Could you check a few things on this model? Use its own coordinates, in mm. Face numbers are marked on the shaded views. A direction names the side the tool comes from. Coordinates: 2 decimals unless noted, no trailing zeros. Write each loop counter-clockwise with the first axis right and the second up, starting at its lowest first coordinate (ties: lowest second). Pieces come first, ordered by that corner, then holes. Notation, with made-up numbers: (66, -7.75) - (111, -7.75) arc R27 ccw to (111, 11.25) - close; hole circle Ø8 at (-21.5, 89). An arc over 180 degrees is marked (long way). Write item = value, one per line. Start each with the question number.
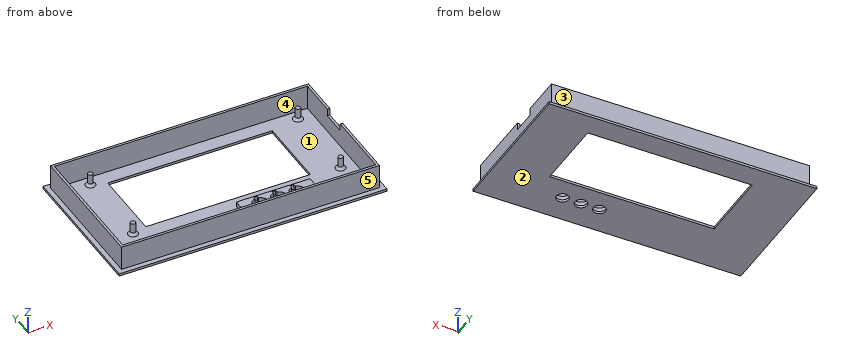
```python
from build123d import *

# Parameters (mm, degrees)
SKETCH015_W     = 109
SKETCH015_H     = 59
SKETCH015_R     = 2.5
SKETCH015_W_2   = 67
SKETCH015_H_2   = 29.5
PAD008_DEPTH    = 1
SKETCH016_R     = 1
PAD009_DEPTH    = 5
SKETCH017_W     = 105
SKETCH017_H     = 55
SKETCH017_W_2   = 103
SKETCH017_H_2   = 53
PAD010_DEPTH    = 10
SKETCH018_W     = 10
SKETCH018_H     = 3
POCKET002_DEPTH = 5
SKETCH019_W     = 30
SKETCH019_H     = 10
PAD011_DEPTH    = 2
CHAMFER008_SIZE = 1


with BuildPart() as part:
    # Sketch015 → Pad008 (new body)
    with BuildSketch(Plane.XY):
        with Locations((54.5, 29.5)):
            Rectangle(SKETCH015_W, SKETCH015_H)
        with Locations((63.6, 11.5)):
            Circle(SKETCH015_R, mode=Mode.SUBTRACT)
        with Locations((71.1, 11.5)):
            Circle(SKETCH015_R, mode=Mode.SUBTRACT)
        with Locations((78.6, 11.5)):
            Circle(SKETCH015_R, mode=Mode.SUBTRACT)
        with Locations((55.1, 35.25)):
            Rectangle(SKETCH015_W_2, SKETCH015_H_2, mode=Mode.SUBTRACT)
    extrude(amount=PAD008_DEPTH)

    # Sketch016 → Pad009 (join)
    with BuildSketch(Plane.XY.offset(1)):
        with Locations((15.6, 52)):
            Circle(SKETCH016_R)
        with Locations((100.1, 52)):
            Circle(SKETCH016_R)
        with Locations((100.1, 19)):
            Circle(SKETCH016_R)
        with Locations((15.6, 19)):
            Circle(SKETCH016_R)
    extrude(amount=PAD009_DEPTH)

    # Sketch017 → Pad010 (join)
    with BuildSketch(Plane.XY.offset(1)):
        with Locations((54.5, 29.5)):
            Rectangle(SKETCH017_W, SKETCH017_H)
        with Locations((54.5, 29.5)):
            Rectangle(SKETCH017_W_2, SKETCH017_H_2, mode=Mode.SUBTRACT)
    extrude(amount=PAD010_DEPTH)

    # Sketch018 (on Face16 of Pad010) → Pocket002 (cut)
    with BuildSketch(Plane.YZ.offset(107)):
        with Locations((35.5, 9.5)):
            Rectangle(SKETCH018_W, SKETCH018_H)
    extrude(amount=-POCKET002_DEPTH, mode=Mode.SUBTRACT)

    # Sketch019 (on Face18 of Pocket002) → Pad011 (join)
    with BuildSketch(Plane.XY.offset(1)):
        with Locations((71.1, 11)):
            Rectangle(SKETCH019_W, SKETCH019_H)
        with BuildLine():
            ThreePointArc((62.85, 14.507906), (63.6, 8.4), (64.35, 14.507906))
            Line((64.35, 15.507906), (64.35, 14.507906))
            Line((62.85, 15.507906), (64.35, 15.507906))
            Line((62.85, 14.507906), (62.85, 15.507906))
        make_face(mode=Mode.SUBTRACT)
        with BuildLine():
            ThreePointArc((70.35, 14.507906), (71.1, 8.4), (71.85, 14.507906))
            Line((71.85, 15.507906), (71.85, 14.507906))
            Line((70.35, 15.507906), (71.85, 15.507906))
            Line((70.35, 14.507906), (70.35, 15.507906))
        make_face(mode=Mode.SUBTRACT)
        with BuildLine():
            ThreePointArc((77.85, 14.507906), (78.6, 8.4), (79.35, 14.507906))
            Line((79.35, 15.507906), (79.35, 14.507906))
            Line((77.85, 15.507906), (79.35, 15.507906))
            Line((77.85, 14.507906), (77.85, 15.507906))
        make_face(mode=Mode.SUBTRACT)
    extrude(amount=PAD011_DEPTH)

    # Chamfer008
    chamfer008_edges = [part.edges().sort_by_distance(p)[0] for p in [
        (14.6, 52, 1),
        (14.6, 19, 1),
        (99.1, 19, 1),
        (99.1, 52, 1),
    ]]
    chamfer(chamfer008_edges, length=CHAMFER008_SIZE)


solid = part.part
```
1) Suppose I cut it at A-A on y = 39. Please give me the cut outline in (x, z), plus the area to 3 significant figures.
2) For P1, Ø4, axis at y = 7.5, z = 7.5, coming from the +X side; P2, Ø1, axis at x = 15.5, y = 18.5, coming from the +Z side; P3, Ø1.5, axis at x = 68.5, y = 48.5, coming from the -Z side; P4, Ø1.1, axis at x = 106.5, z = 10, coming from the +Y side, each with a flat end and sliding along its axis, tell me the tip position at first contact or that it passes through.
3) If I drill on probe 1 along Y at (x, z) = (71.1, 2.65); probe 2 along Y at (x, z) = (78.6, 0.85); probe 3 along X at (y, z) = (11.5, 1.65), over which ranges is the centre line in solid material (lowest first)? Write a range as [from, to].
4) Which directions (+Z, -Z, +X, -X, +Y, -Y) give clear straight access to the entire face, cutting with the end or side of a thin tool? Please do the marked faces 3, 4 and 5.
5) Suppose I cut it at D-D on y = 52. Please give me the cut outline in (x, z), plus the area to 3 significant figures.
6) Suppose I cut it at B-B on x = 38. Please give me the cut outline in (y, z).
7) Suppose I cut it at C-C on z = 4.5. Please give me the cut outline in (x, y).
8) Thinking about a two-plate mould opening in X: for the marked faces 1 and 2, which applies, +X half, -X half, draft (parallel to the pull), parting line (faces both ways), or undercut?
Reply:
q1.outline = (0, 0) - (21.6, 0) - (21.6, 1) - (3, 1) - (3, 11) - (2, 11) - (2, 1) - (0, 1) - close; (88.6, 0) - (109, 0) - (109, 1) - (107, 1) - (107, 8) - (106, 8) - (106, 1) - (88.6, 1) - close
q1.area = 59.0 mm^2
q2.P1 = 107
q2.P2 = 6
q2.P3 = through
q2.P4 = 57
q3.probe_1 = [2, 3], [6, 8.4], [15.51, 16], [56, 57]
q3.probe_2 = [0, 9], [14, 20.5], [50, 59]
q3.probe_3 = [2, 3], [56.1, 60.5], [66.7, 68], [74.2, 75.5], [81.7, 86.1], [106, 107]
q4.face_3 = +Z, +X, -X, +Y
q4.face_4 = +Z
q4.face_5 = +Z, +X, -X, -Y
q5.outline = (0, 0) - (109, 0) - (109, 1) - (107, 1) - (107, 11) - (106, 11) - (106, 1) - (102.1, 1) - (101.1, 2) - (101.1, 6) - (99.1, 6) - (99.1, 2) - (98.1, 1) - (17.6, 1) - (16.6, 2) - (16.6, 6) - (14.6, 6) - (14.6, 2) - (13.6, 1) - (3, 1) - (3, 11) - (2, 11) - (2, 1) - (0, 1) - close
q5.area = 151 mm^2
q6.outline = (0, 0) - (20.5, 0) - (20.5, 1) - (3, 1) - (3, 11) - (2, 11) - (2, 1) - (0, 1) - close; (50, 0) - (59, 0) - (59, 1) - (57, 1) - (57, 11) - (56, 11) - (56, 1) - (50, 1) - close
q7.outline = (2, 2) - (107, 2) - (107, 57) - (2, 57) - close; circle Ø2 at (15.6, 19); circle Ø2 at (15.6, 52); circle Ø2 at (100.1, 19); circle Ø2 at (100.1, 52); hole (3, 3) - (106, 3) - (106, 56) - (3, 56) - close
q8.face_1 = undercut
q8.face_2 = draft
